```python
from build123d import *

# Parameters (mm, degrees)
SKETCH1_W           = 16.26
SKETCH1_H           = 16.26
SKETCH1_W_2         = 4.1
SKETCH1_H_2         = 3
BOSS_EXTRUDE1_DEPTH = 1.6
SKETCH1_3_W         = 4.1
SKETCH1_3_H         = 3
BOSS_EXTRUDE2_DEPTH = 7.1
SKETCH2_R           = 2.05
CUT_EXTRUDE1_DEPTH  = 24.643713752
SKETCH3_W           = 7.5
SKETCH3_H           = 3
BOSS_EXTRUDE3_DEPTH = 6.5


with BuildPart() as part:
    # Sketch1 → Boss-Extrude1 (new body)
    # profile 1 of 2: a face of its own
    with BuildSketch(Plane(origin=(0, 0, 0), x_dir=(0, 0, -1), z_dir=(1, 0, 0))):
        with Locations((8.13, -8.13)):
            Rectangle(SKETCH1_W, SKETCH1_H)
        with Locations((4.33, -1.8)):
            Rectangle(SKETCH1_W_2, SKETCH1_H_2, mode=Mode.SUBTRACT)
    # profile 2 of 2: a face of its own
    with BuildSketch(Plane(origin=(0, 0, 0), x_dir=(0, 0, -1), z_dir=(1, 0, 0))):
        with Locations((4.33, -1.8)):
            Rectangle(SKETCH1_W_2, SKETCH1_H_2)
    extrude(amount=BOSS_EXTRUDE1_DEPTH)

    # Sketch1_3 → Boss-Extrude2 (add)
    with BuildSketch(Plane(origin=(0, 0, 0), x_dir=(0, 0, -1), z_dir=(1, 0, 0))):
        with Locations((4.33, -1.8)):
            Rectangle(SKETCH1_3_W, SKETCH1_3_H)
    extrude(amount=BOSS_EXTRUDE2_DEPTH)

    # Sketch2 → Cut-Extrude1 (cut, through all)
    with BuildSketch(Plane(origin=(1.6, 0, 0), x_dir=(0, 0, -1), z_dir=(1, 0, 0))):
        with Locations((11.47, -4.58)):
            Circle(SKETCH2_R)
    extrude(amount=-CUT_EXTRUDE1_DEPTH, mode=Mode.SUBTRACT)

    # Sketch3 → Boss-Extrude3 (add)
    with BuildSketch(Plane(origin=(1.6, 0, 0), x_dir=(0, 0, -1), z_dir=(1, 0, 0))):
        with Locations((5.75, -12.76)):
            Rectangle(SKETCH3_W, SKETCH3_H)
    extrude(amount=-BOSS_EXTRUDE3_DEPTH)


solid = part.part
```
Design review of the part built by this model. Coordinates are the model's own, in mm. A direction names the side the tool comes from. Give positions to 0.01 mm unless a question says otherwise; leave off trailing zeros. Loops run counter-clockwise (first coordinate to the right, second up) from the corner with the lowest first, then second, coordinate; pieces in that order, holes last. Notation, with made-up numbers: M -19,87 L 8,87 A16 cw 8,112 Z; hole C 78,54 d11. An arc over 180 degrees is marked long. Return JSON: item names as keys, results as strings. Group by question number.
Item 1: Insertion check: pin 1 Ø3.5 at (x, y) = (4, -2.5) entering from +Z; pin 2 Ø4.5 at (x, z) = (5, -5) entering from -Y; pin 3 Ø3.5 at (x, z) = (5.5, -4) entering from +Y. Each pin has a flat end and moves straight along its axis. Give the tip position at first contact, or say it passes through.
Item 2: We need section A-A (y = -4.58). Give the boundary of the cut face in (x, z).
Item 3: We need section D-D (y = -12.75). Give the boundary of the cut face in (x, z), and give its area (3 significant figures).
Item 4: Tool access review of faces 1 (the flat face through (4, -2, -2.28)), 2 (the flat face through (-2, -14.26, -6)), 3 (the flat face through (-2, -13, -9.5)): name each direction out of +Z, -Z, +X, -X, +Y, -Y from which nothing blocks a thin tool from reaching the whole face with its end or side.
Item 5: We need section C-C (z = -7). Give the boundary of the cut face in (x, y).
Item 6: We need section B-B (z = -11.47). Give the boundary of the cut face in (x, y), and give its area (3 significant figures).
Item 7: For probe 1 along X at (y, z) = (-11.5, -5.5); probe 2 along X at (y, z) = (-4.75, -7.75); probe 3 along Y at (x, z) = (1.05, -11.47), list the stretches that pass through material, from the lowest coordinate up.
Output:
{
 "1": {"pin 1": "stops at z = -2.28", "pin 2": "stops at y = -3.3", "pin 3": "stops at y = -0.3"},
 "2": {"outline": "M 0,-16.26 L 1.6,-16.26 L 1.6,-13.52 L 0,-13.52 Z; M 0,-9.42 L 1.6,-9.42 L 1.6,0 L 0,0 Z"},
 "3": {"outline": "M -4.9,-9.5 L 0,-9.5 L 0,-16.26 L 1.6,-16.26 L 1.6,0 L 0,0 L 0,-2 L -4.9,-2 Z", "area": "62.8 mm^2"},
 "4": {"face 1": "+Z, +X, +Y, -Y", "face 2": "+Z, -Z, -X, -Y", "face 3": "-Z, -X, +Y, -Y"},
 "5": {"outline": "M -4.9,-14.26 L 0,-14.26 L 0,-16.26 L 1.6,-16.26 L 1.6,0 L 0,0 L 0,-11.26 L -4.9,-11.26 Z"},
 "6": {"outline": "M 0,-16.26 L 1.6,-16.26 L 1.6,-6.63 L 0,-6.63 Z; M 0,-2.53 L 1.6,-2.53 L 1.6,0 L 0,0 Z", "area": "19.5 mm^2"},
 "7": {"probe 1": "x = -4.9 to 1.6", "probe 2": "x = 0 to 1.6", "probe 3": "y = -16.26 to -6.63, -2.53 to 0"}
}
